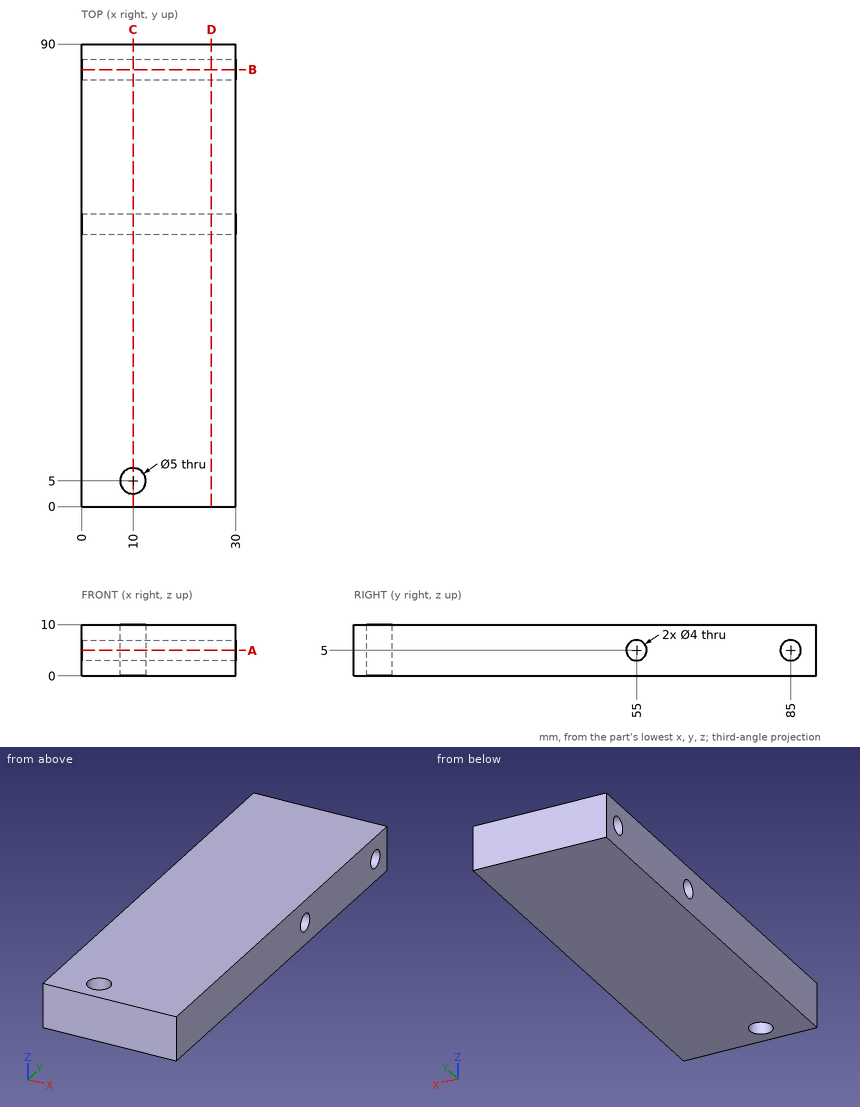
Here's the drawing with two shaded views (mm, measured from the low corner). I have some questions. Give positions to 0.01 mm unless a question says otherwise; leave off trailing zeros. Order: outer loops, then holes, each group sorted by start corner. A loop starts at its lowest first (then second) coordinate and runs counter-clockwise, first axis right, second up. Notation, with made-up numbers: (84, 88.25) -> (134, 88.25) arc R23 cw to (134, 99.25) -> close; hole circle Ø4 at (47.5, 51). An arc over 180 degrees is marked (long way). One line per item, written item: value. Start each with the question number.
1. Imagine slicing it at B-B, the plane y = 85. List the corners of the cut face in (x, z) for me.
2. Will this pin go through, and if not, where does the flat tip stop? pin 1 Ø3 at (y, z) = (85, 5) entering from +X.
3. Imagine slicing it at D-D, the plane x = 25.25. List the corners of the cut face in (y, z) for me, plus the area to 3 significant figures.
4. Imagine slicing it at C-C, the plane x = 10. List the corners of the cut face in (y, z) for me.
5. Imagine slicing it at A-A, the plane z = 5. List the corners of the cut face in (x, y) for me.
6. I need wall thicknesses on probe 1 along Y at (x, z) = (16, 5); probe 2 along Y at (x, z) = (10, 7.25); probe 3 along Y at (x, z) = (6.25, 4). Which ranges of each line are inside material? Lowest first, please. Write a range as from..to.
Values follow:
1. outline: (0, 0) -> (30, 0) -> (30, 3) -> (0, 3) -> close; (0, 7) -> (30, 7) -> (30, 10) -> (0, 10) -> close
2. pin 1: passes through
3. outline: (0, 0) -> (90, 0) -> (90, 10) -> (0, 10) -> close; hole circle Ø4 at (55, 5); hole circle Ø4 at (85, 5)
3. area: 875 mm2
4. outline: (0, 0) -> (2.5, 0) -> (2.5, 10) -> (0, 10) -> close; (7.5, 0) -> (90, 0) -> (90, 10) -> (7.5, 10) -> close; hole circle Ø4 at (55, 5); hole circle Ø4 at (85, 5)
5. outline: (0, 0) -> (30, 0) -> (30, 53) -> (0, 53) -> close; (0, 57) -> (30, 57) -> (30, 83) -> (0, 83) -> close; (0, 87) -> (30, 87) -> (30, 90) -> (0, 90) -> close; hole circle Ø5 at (10, 5)
6. probe 1: y = 0..53, 57..83, 87..90
6. probe 2: y = 0..2.5, 7.5..90
6. probe 3: y = 0..53.27, 56.73..83.27, 86.73..90
